Geometry: final body of the model. Coordinates: model frame, mm. Round coordinates to 2 decimals unless told otherwise and drop trailing zeros. Loops run counter-clockwise (first coordinate to the right, second up) from the corner with the lowest first, then second, coordinate; pieces in that order, holes last. Notation, with made-up numbers: (32, 37.5) -> (74, 37.5) arc R4 cw to (74, 41.5) -> close; hole circle Ø5 at (-21.75, 81). An arc over 180 degrees is marked (long way). Answer in a Markdown table with one row per item.
```python
from build123d import *

# Parameters (mm, degrees)
SKETCH2_R           = 1.5
SKETCH2_R_2         = 4
BOSS_EXTRUDE1_DEPTH = 5


with BuildPart() as part:
    # Sketch2 → Boss-Extrude1 (new body)
    with BuildSketch(Plane(origin=(0, 0, 0), x_dir=(0, 0, -1), z_dir=(1, 0, 0))):
        with BuildLine():
            Line((92.352467742, 33.761940445), (60.516758506, 62.666743117))
            ThreePointArc((60.516758506, 62.666743117), (61.485484965, 61.324652748), (61.827939653, 59.705281792))
            ThreePointArc((61.827939653, 59.705281792), (59.447310609, 56.047736481), (55.1391208, 56.743820468))
            Line((55.1391208, 56.743820468), (86.974830036, 27.839017797))
            ThreePointArc((86.974830036, 27.839017797), (86.702187565, 33.489297974), (92.352467742, 33.761940445))
        make_face()
        with Locations((69.679349119, 48.944954468)):
            Circle(SKETCH2_R, mode=Mode.SUBTRACT)
        with Locations((57.827939653, 59.705281792)):
            Circle(SKETCH2_R_2)
        with Locations((57.827939653, 59.705281792)):
            Circle(SKETCH2_R, mode=Mode.SUBTRACT)
        with Locations((89.663648889, 30.800479121)):
            Circle(SKETCH2_R_2)
        with Locations((89.663648889, 30.800479121)):
            Circle(SKETCH2_R, mode=Mode.SUBTRACT)
    extrude(amount=BOSS_EXTRUDE1_DEPTH)


solid = part.part
```
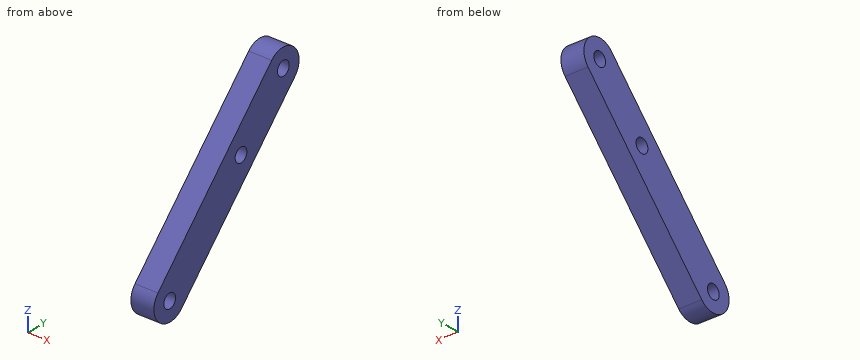
Item 1: Section query C-C, the plane y = 30. Output: boundary loops of the cut face in (x, z).
Ans:
| item | result |
|---|---|
| outline | (0, -93.58) -> (5, -93.58) -> (5, -90.93) -> (0, -90.93) -> close; (0, -88.4) -> (5, -88.4) -> (5, -84.59) -> (0, -84.59) -> close |
Item 2: Ray query, L1, parallel to Y at x = 2, z = -91; L2, parallel to Y at x = 1.6, z = -57; L3, parallel to Y at x = 3.9, z = -75. Return the intervals inside material, ascending.
Ans:
| item | result |
|---|---|
| L1 | 27.03 to 30.12, 31.48 to 34.99 |
| L2 | 55.05 to 58.45, 60.96 to 63.62 |
| L3 | 38.71 to 49.52 |
Item 3: Section query D-D, the plane z = -77.5. Output: boundary loops of the cut face in (x, y).
Ans:
| item | result |
|---|---|
| outline | (0, 36.44) -> (5, 36.44) -> (5, 47.25) -> (0, 47.25) -> close |
Item 4: Section query B-B, the plane x = 1.35. Output: boundary loops of the cut face in (y, z), and give its area (3 significant figures).
Ans:
| item | result |
|---|---|
| outline | (27.84, -86.97) arc R4 ccw to (33.76, -92.35) -> (62.67, -60.52) arc R4 ccw to (56.74, -55.14) -> close; hole circle Ø3 at (30.8, -89.66); hole circle Ø3 at (48.94, -69.68); hole circle Ø3 at (59.71, -57.83) |
| area | 373 mm2 |
Item 5: Section query A-A, the plane y = 59. Output: boundary loops of the cut face in (x, z).
Ans:
| item | result |
|---|---|
| outline | (0, -64.56) -> (5, -64.56) -> (5, -59.15) -> (0, -59.15) -> close; (0, -56.5) -> (5, -56.5) -> (5, -53.89) -> (0, -53.89) -> close |
Item 6: First-contact query: P1, Ø3, axis at x = 4, y = 40.5, coming from the -Z side; P2, Ø3, axis at x = 3.5, y = 33.5, coming from the -Z side; P3, Ø1.5, axis at x = 1, z = -80, coming from the -Y side. Flat tips, straight axial feed; report the tip coordinate or a pass-through.
Ans:
| item | result |
|---|---|
| P1 | z = -86.58 |
| P2 | z = -93.48 |
| P3 | y = 33.49 |
